Source: CAD feature listing. Evaluate the final solid. Frame: model axes, mm. Give positions to 0.01 mm unless a question says otherwise; leave off trailing zeros. Order: outer loops, then holes, each group sorted by start corner. A loop starts at its lowest first (then second) coordinate and runs counter-clockwise, first axis right, second up.
1) Section A-A, the plane x = 243. Return loops of the section in (y, z) (3 decimals).
2) Material intervals for line 1 (Z direction, x = 297, y = -1.25) (3 decimals); line 2 (X direction, y = -1, z = 76) (3 decimals); line 3 (X direction, y = -1, z = 68.5) (3 decimals), sorted ascending.
3) Section B-B, the plane x = 528. Return loops of the section in (y, z).
4) First-contact query: P1, Ø0.5, axis at x = 956, y = -0.5, coming from the +Z side; P2, Ø0.8, axis at x = 233, y = -1, coming from the +Z side (3 decimals); P3, Ø0.8, axis at y = -1, z = 89.5, coming from the -X side. Flat tips, straight axial feed; report the tip coordinate or a pass-through.
5) Section D-D, the plane x = 733. Return loops of the section in (y, z), plus the area to 3 significant figures.
6) Section C-C, the plane y = -0.25. Give the number of separate pieces and of enclosed holes in the cut face, plus the area to 3 significant figures.
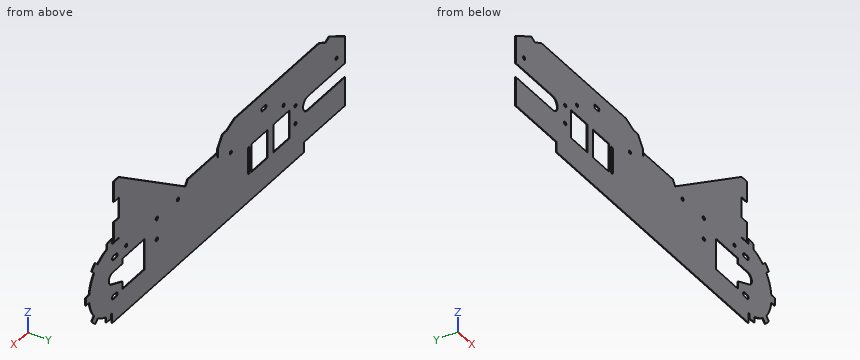
```python
from build123d import *

# Parameters (mm, degrees)
F0_R     = 4.1275
F0_W     = 60.325
F0_H     = 69.85
F0_R_2   = 4.318
F0_R_3   = 4.0005
F0_W_2   = 19.05
F0_H_2   = 50.8
F0_W_3   = 714.375
F0_H_3   = 25.4
F1_DEPTH = 1.5748
F2_W     = 19.05
F2_H     = 1.5748
F3_DEPTH = 25.4


with BuildPart() as f1:
    # F0 (on Front) → F1 (new body)
    with BuildSketch(Plane.XZ):
        with BuildLine():
            Line((0, 71.12), (0, 0))
            Line((0, 0), (152.4, 0))
            Line((152.4, 0), (866.775, 0))
            ThreePointArc((866.775, 0), (868.892405, 0.026154), (871.008518, 0.1046))
            ThreePointArc((871.008518, 0.1046), (880.495682, 1.105153), (889.812929, 3.15364))
            ThreePointArc((889.812929, 3.15364), (905.833291, 9.414938), (920.281197, 18.748418))
            ThreePointArc((920.281197, 18.748418), (923.925, 21.829358), (927.391729, 25.108271))
            Line((927.391729, 25.108271), (876.016834, 76.483166))
            ThreePointArc((876.016834, 76.483166), (873.488274, 74.143986), (870.473354, 72.477963))
            Line((870.473354, 72.477963), (828.60841, 55.5625))
            Line((828.60841, 55.5625), (828.60841, 36.5125))
            Line((828.60841, 36.5125), (746.05841, 36.5125))
            Line((746.05841, 36.5125), (746.05841, 112.7125))
            Line((746.05841, 112.7125), (828.60841, 112.7125))
            Line((828.60841, 112.7125), (828.60841, 100.0125))
            Line((828.60841, 100.0125), (865.12091, 100.0125))
            ThreePointArc((865.12091, 100.0125), (871.124657, 98.689863), (876.016834, 94.966834))
            Line((876.016834, 94.966834), (927.391729, 146.341729))
            ThreePointArc((927.391729, 146.341729), (923.925, 149.620642), (920.281197, 152.701582))
            ThreePointArc((920.281197, 152.701582), (903.936518, 162.976519), (885.707042, 169.333333))
            ThreePointArc((885.707042, 169.333333), (876.3, 170.91919), (866.775, 171.45))
            Line((866.775, 171.45), (860.425, 171.45))
            Line((860.425, 171.45), (841.375, 171.45))
            Line((841.375, 171.45), (841.375, 222.25))
            Line((841.375, 222.25), (841.375, 273.05))
            Line((841.375, 273.05), (841.375, 323.85))
            Line((841.375, 323.85), (593.725, 152.4))
            Line((593.725, 152.4), (473.075, 152.4))
            Line((473.075, 152.4), (439.727616, 200.025))
            Line((439.727616, 200.025), (71.490397, 200.025))
            Line((71.490397, 200.025), (0, 158.75))
            Line((0, 158.75), (0, 106.045))
            Line((0, 106.045), (138.1125, 106.045))
            ThreePointArc((138.1125, 106.045), (155.575, 88.5825), (138.1125, 71.12))
            Line((138.1125, 71.12), (0, 71.12))
        make_face()
        with Locations((184.0865, 65.0875)):
            Circle(F0_R, mode=Mode.SUBTRACT)
        Polygon((206.375, 41.91), (206.375, 88.5825), (206.375, 111.76), (266.7, 111.76), (266.7, 41.91), align=None, mode=Mode.SUBTRACT)
        with BuildLine():
            ThreePointArc((27.305, 136.9695), (31.3055, 140.97), (35.306, 136.9695))
            ThreePointArc((35.306, 136.9695), (31.3055, 132.969), (27.305, 136.9695))
        make_face(mode=Mode.SUBTRACT)
        with Locations((184.0865, 109.8169)):
            Circle(F0_R, mode=Mode.SUBTRACT)
        with BuildLine():
            ThreePointArc((224.0788, 136.9695), (228.0793, 140.97), (232.0798, 136.9695))
            ThreePointArc((232.0798, 136.9695), (228.0793, 132.969), (224.0788, 136.9695))
        make_face(mode=Mode.SUBTRACT)
        with Locations((317.9445, 76.835)):
            Rectangle(F0_W, F0_H, mode=Mode.SUBTRACT)
        with BuildLine():
            ThreePointArc((361.599438, 47.166166), (358.077275, 43.497828), (354.457, 47.069375))
            Line((354.457, 47.069375), (354.457, 106.600625))
            ThreePointArc((354.457, 106.600625), (357.980475, 110.172172), (361.599438, 106.697416))
            ThreePointArc((361.599438, 106.697416), (361.60075, 106.600625), (361.599438, 106.503834))
            Line((361.599438, 106.503834), (361.599438, 47.166166))
        make_face(mode=Mode.SUBTRACT)
        with BuildLine():
            ThreePointArc((428.8536, 136.9695), (424.8531, 132.969), (420.8526, 136.9695))
            ThreePointArc((420.8526, 136.9695), (424.8531, 140.97), (428.8536, 136.9695))
        make_face(mode=Mode.SUBTRACT)
        with BuildLine():
            ThreePointArc((852.03991, 31.8008), (846.89641, 36.9443), (852.03991, 42.0878))
            Line((852.03991, 42.0878), (862.32691, 42.0878))
            ThreePointArc((862.32691, 42.0878), (865.963914, 40.581304), (867.47041, 36.9443))
            ThreePointArc((867.47041, 36.9443), (865.963914, 33.307296), (862.32691, 31.8008))
            Line((862.32691, 31.8008), (852.03991, 31.8008))
        make_face(mode=Mode.SUBTRACT)
        with Locations((700.59241, 84.5185)):
            Circle(F0_R_2, mode=Mode.SUBTRACT)
        with BuildLine():
            ThreePointArc((625.6274, 136.9695), (621.6269, 132.969), (617.6264, 136.9695))
            ThreePointArc((617.6264, 136.9695), (621.6269, 140.97), (625.6274, 136.9695))
        make_face(mode=Mode.SUBTRACT)
        with Locations((700.59241, 136.5885)):
            Circle(F0_R_2, mode=Mode.SUBTRACT)
        with Locations((814.70191, 137.033)):
            Circle(F0_R_3, mode=Mode.SUBTRACT)
        with BuildLine():
            ThreePointArc((852.03991, 129.2225), (846.89641, 134.366), (852.03991, 139.5095))
            Line((852.03991, 139.5095), (862.32691, 139.5095))
            ThreePointArc((862.32691, 139.5095), (865.963914, 138.003004), (867.47041, 134.366))
            ThreePointArc((867.47041, 134.366), (865.963914, 130.728996), (862.32691, 129.2225))
            Line((862.32691, 129.2225), (852.03991, 129.2225))
        make_face(mode=Mode.SUBTRACT)
        with BuildLine():
            ThreePointArc((306.451, 178.562), (309.773695, 177.185695), (311.15, 173.863))
            ThreePointArc((311.15, 173.863), (309.773695, 170.540305), (306.451, 169.164))
            Line((306.451, 169.164), (297.053, 169.164))
            ThreePointArc((297.053, 169.164), (292.354, 173.863), (297.053, 178.562))
            Line((297.053, 178.562), (306.451, 178.562))
        make_face(mode=Mode.SUBTRACT)
        with BuildLine():
            ThreePointArc((876.016834, 94.966834), (878.533743, 90.647253), (879.40841, 85.725))
            Line((879.40841, 85.725), (952.5, 85.725))
            ThreePointArc((952.5, 85.725), (952.367195, 90.49489), (951.96919, 95.25))
            ThreePointArc((951.96919, 95.25), (945.974573, 118.530537), (933.751582, 139.231197))
            ThreePointArc((933.751582, 139.231197), (930.670642, 142.875), (927.391729, 146.341729))
            Line((927.391729, 146.341729), (876.016834, 94.966834))
        make_face()
        with BuildLine():
            Line((876.016834, 76.483166), (927.391729, 25.108271))
            ThreePointArc((927.391729, 25.108271), (930.670642, 28.575), (933.751582, 32.218803))
            ThreePointArc((933.751582, 32.218803), (945.974573, 52.919463), (951.96919, 76.2))
            ThreePointArc((951.96919, 76.2), (952.367195, 80.95511), (952.5, 85.725))
            Line((952.5, 85.725), (879.40841, 85.725))
            ThreePointArc((879.40841, 85.725), (878.533743, 80.802747), (876.016834, 76.483166))
        make_face()
        with BuildLine():
            ThreePointArc((866.775, 171.45), (876.3, 170.91919), (885.707042, 169.333333))
            Line((885.707042, 169.333333), (885.735586, 182.306452))
            ThreePointArc((885.735586, 182.306452), (876.3, 183.688029), (866.775, 184.15))
            Line((866.775, 184.15), (866.775, 171.45))
        make_face()
        with Locations((850.9, 196.85)):
            Rectangle(F0_W_2, F0_H_2)
        with Locations((850.9, 298.45)):
            Rectangle(F0_W_2, F0_H_2)
        with BuildLine():
            ThreePointArc((920.281197, 152.701582), (923.925, 149.620642), (927.391729, 146.341729))
            Line((927.391729, 146.341729), (936.371985, 155.321985))
            ThreePointArc((936.371985, 155.321985), (932.918717, 158.611826), (929.31013, 161.730514))
            Line((929.31013, 161.730514), (920.281197, 152.701582))
        make_face()
        with BuildLine():
            Line((936.371985, 155.321985), (927.391729, 146.341729))
            ThreePointArc((927.391729, 146.341729), (930.670642, 142.875), (933.751582, 139.231197))
            Line((933.751582, 139.231197), (942.780514, 148.26013))
            ThreePointArc((942.780514, 148.26013), (939.661826, 151.868717), (936.371985, 155.321985))
        make_face()
        with BuildLine():
            ThreePointArc((951.96919, 95.25), (952.367195, 90.49489), (952.5, 85.725))
            Line((952.5, 85.725), (965.2, 85.725))
            Line((965.2, 85.725), (964.738029, 95.25))
            Line((964.738029, 95.25), (951.96919, 95.25))
        make_face()
        with BuildLine():
            ThreePointArc((952.5, 85.725), (952.367195, 80.95511), (951.96919, 76.2))
            Line((951.96919, 76.2), (964.738029, 76.2))
            ThreePointArc((964.738029, 76.2), (965.084439, 80.956902), (965.2, 85.725))
            Line((965.2, 85.725), (952.5, 85.725))
        make_face()
        with BuildLine():
            ThreePointArc((933.751582, 32.218803), (930.670642, 28.575), (927.391729, 25.108271))
            Line((927.391729, 25.108271), (936.371985, 16.128015))
            ThreePointArc((936.371985, 16.128015), (939.661826, 19.581283), (942.780514, 23.18987))
            Line((942.780514, 23.18987), (933.751582, 32.218803))
        make_face()
        with BuildLine():
            ThreePointArc((927.391729, 25.108271), (923.925, 21.829358), (920.281197, 18.748418))
            Line((920.281197, 18.748418), (929.31013, 9.719486))
            ThreePointArc((929.31013, 9.719486), (932.918717, 12.838174), (936.371985, 16.128015))
            Line((936.371985, 16.128015), (927.391729, 25.108271))
        make_face()
        with BuildLine():
            ThreePointArc((889.812929, 3.15364), (880.495682, 1.105153), (871.008518, 0.1046))
            Line((871.008518, 0.1046), (871.008518, -12.60891))
            ThreePointArc((871.008518, -12.60891), (880.504832, -11.737671), (889.872261, -9.951524))
            Line((889.872261, -9.951524), (889.812929, 3.15364))
        make_face()
        with Locations((509.5875, -12.7)):
            Rectangle(F0_W_3, F0_H_3)
        Polygon((478.149444, 165.1), (473.075, 152.4), (593.725, 152.4), (584.932692, 165.1), align=None)
        Polygon((455.231453, 200.025), (439.727616, 200.025), (473.075, 152.4), (473.075, 174.541774), align=None)
        Polygon((95.536456, 212.725), (71.490397, 200.025), (439.727616, 200.025), (410.032392, 212.725), align=None)
        Polygon((0, 173.414697), (0, 158.75), (71.490397, 200.025), (57.889698, 206.837329), align=None)
    extrude(amount=F1_DEPTH)

    # F2 (on face) → F3 (cut)
    with BuildSketch(Plane.XZ.offset(1.5748)):
        with Locations((850.9, 172.2374)):
            Rectangle(F2_W, F2_H)
    extrude(amount=-F3_DEPTH, mode=Mode.SUBTRACT)


solid = f1.part
```
From the geometry:
1. outline: (-1.575, -25.4) - (0, -25.4) - (0, 41.91) - (-1.575, 41.91) - close; (-1.575, 111.76) - (0, 111.76) - (0, 212.725) - (-1.575, 212.725) - close
2. line 1: z = -25.4 to 41.91, 111.76 to 169.164, 178.562 to 212.725
2. line 2: x = 150.221 to 206.375, 266.7 to 287.782, 348.107 to 354.457, 361.599 to 746.058, 875.588 to 951.947
2. line 3: x = 0 to 181.765, 186.408 to 206.375, 266.7 to 287.782, 348.107 to 354.457, 361.599 to 746.058, 860.628 to 950.752
3. outline: (-1.57, -25.4) - (0, -25.4) - (0, 165.1) - (-1.57, 165.1) - close
4. P1: stops at z = 95.25
4. P2: stops at z = 212.725
4. P3: stops at x = 155.53
5. outline: (-1.57, -25.4) - (0, -25.4) - (0, 248.82) - (-1.57, 248.82) - close
5. area: 432 mm2
6. separate pieces: 1
6. enclosed holes: 16
6. area: 191,000 mm2
